from build123d import *

# Parameters (mm, degrees)
SKETCH1_R           = 12.3
BOSS_EXTRUDE1_DEPTH = 24.5
SKETCH2_R           = 8.9
CUT_EXTRUDE1_DEPTH  = 20
SKETCH3_R           = 7.4
CUT_EXTRUDE2_DEPTH  = 1
SKETCH4_R           = 4.5
CUT_EXTRUDE3_DEPTH  = 30.237475951


with BuildPart() as part:
    # Sketch1 → Boss-Extrude1 (new body)
    with BuildSketch(Plane(origin=(0, 0, 0), x_dir=(1, 0, 0), z_dir=(0, 1, 0))):
        with Locations(Location((0, 0, 0), (0, 0, 270))):
            Circle(SKETCH1_R)
    extrude(amount=BOSS_EXTRUDE1_DEPTH)

    # Sketch2 → Cut-Extrude1 (cut)
    with BuildSketch(Plane(origin=(0, 24.5, 0), x_dir=(1, 0, 0), z_dir=(0, 1, 0))):
        with Locations(Location((0, 0, 0), (0, 0, 270))):
            Circle(SKETCH2_R)
    extrude(amount=-CUT_EXTRUDE1_DEPTH, mode=Mode.SUBTRACT)

    # Sketch3 → Cut-Extrude2 (cut)
    with BuildSketch(Plane.XZ):
        with Locations(Location((0, 0, 0), (0, 0, 270))):
            Circle(SKETCH3_R)
    extrude(amount=-CUT_EXTRUDE2_DEPTH, mode=Mode.SUBTRACT)

    # Sketch4 → Cut-Extrude3 (cut, through all)
    with BuildSketch(Plane.XZ.offset(-1)):
        with Locations(Location((0, 0, 0), (0, 0, 270))):
            Circle(SKETCH4_R)
    extrude(amount=-CUT_EXTRUDE3_DEPTH, mode=Mode.SUBTRACT)


solid = part.part
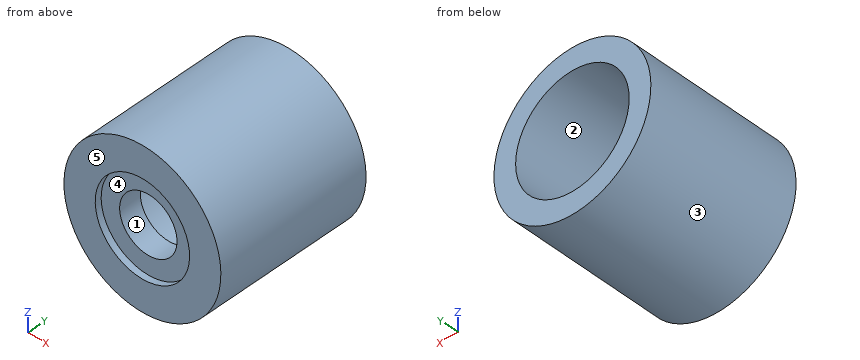
CAD build for the part. Positions are in the model's coordinates, mm. Face numbers are marked on the shaded views. A direction names the side the tool comes from. Round coordinates to 2 decimals unless told otherwise and drop trailing zeros. Write each loop counter-clockwise with the first axis right and the second up, starting at its lowest first coordinate (ties: lowest second). Pieces come first, ordered by that corner, then holes.
(1) Slice it at A-A, the plane x = 0. Write the cut outline in (y, z).
(2) Slice it at B-B, the plane z = 0. Write the cut outline in (x, y).
(3) 3-axis set-ups, long thin cutter, end or side, ignore diameter. For the marked faces 1 and 2: which of +Z, -Z, +X, -X, +Y, -Y reach the whole face in a straight line?
(4) Probe line 1 along X through (y, z) = (0.3, 0); line 2 along X through (y, z) = (3.6, 0); line 3 along Y through (x, z) = (-8.5, 0.5). List the from-to ranges inside material, lowest first.
(5) Slice it at D-D, the plane z = 6.25. Write the cut outline in (x, y).
(6) Drop flat-ended pins along their axis: P1, Ø1, axis at x = -3.5, y = 17.5, coming from the +Z side; P2, Ø10.5, axis at x = 0, z = 0, coming from the +Y side; P3, Ø7.5, axis at x = 3, z = -0.5, coming from the -Y side. Give the stop position or say it passes through.
(7) Mould opens along X. For the marked faces 3, 4 and 5 say: pulls with the +X half, pulls with the -X half, needs draft (parallel to the pull), parting line crosses it, or undercut.
(8) Slice it at C-C, the plane y = 17. Write the cut outline in (x, z).
From the geometry:
1. outline: (0, -12.3) - (24.5, -12.3) - (24.5, -8.9) - (4.5, -8.9) - (4.5, -4.5) - (1, -4.5) - (1, -7.4) - (0, -7.4) - close; (0, 7.4) - (1, 7.4) - (1, 4.5) - (4.5, 4.5) - (4.5, 8.9) - (24.5, 8.9) - (24.5, 12.3) - (0, 12.3) - close
2. outline: (-12.3, 0) - (-7.4, 0) - (-7.4, 1) - (-4.5, 1) - (-4.5, 4.5) - (-8.9, 4.5) - (-8.9, 24.5) - (-12.3, 24.5) - close; (4.5, 1) - (7.4, 1) - (7.4, 0) - (12.3, 0) - (12.3, 24.5) - (8.9, 24.5) - (8.9, 4.5) - (4.5, 4.5) - close
3. face 1: +Y, -Y
3. face 2: +Y
4. line 1: x = -12.3 to -7.4, 7.4 to 12.3
4. line 2: x = -12.3 to -4.5, 4.5 to 12.3
4. line 3: y = 0 to 4.5
5. outline: (-10.59, 0) - (-3.96, 0) - (-3.96, 1) - (3.96, 1) - (3.96, 0) - (10.59, 0) - (10.59, 24.5) - (6.34, 24.5) - (6.34, 4.5) - (-6.34, 4.5) - (-6.34, 24.5) - (-10.59, 24.5) - close
6. P1: stops at z = 11.93
6. P2: stops at y = 4.5
6. P3: stops at y = 1
7. face 3: parting line crosses it
7. face 4: undercut
7. face 5: needs draft
8. outline: circle Ø24.6 at (0, 0); hole circle Ø17.8 at (0, 0)
